```python
from build123d import *

# Parameters (mm, degrees)
SKETCH1_R           = 2.38125
BOSS_EXTRUDE1_DEPTH = 1.5875
SKETCH2_R           = 3.96875
BOSS_EXTRUDE2_DEPTH = 1.5875


with BuildPart() as part:
    # Sketch1 → Boss-Extrude1 (new body)
    with BuildSketch(Plane(origin=(0, 0, 0), x_dir=(1, 0, 0), z_dir=(0, 1, 0))):
        with BuildLine():
            Line((3.96875, 0), (3.921336464, 0.61163461))
            ThreePointArc((3.921336464, 0.61163461), (0, 3.96875), (-3.921336464, 0.61163461))
            Line((-3.921336464, 0.61163461), (-3.96875, 0))
            ThreePointArc((-3.96875, 0), (0, -3.96875), (3.96875, 0))
        make_face()
        with BuildLine():
            Line((3.921336464, 0.61163461), (2.38125, 20.47875))
            ThreePointArc((2.38125, 20.47875), (0, 18.0975), (-2.38125, 20.47875))
            Line((-2.38125, 20.47875), (-3.921336464, 0.61163461))
            ThreePointArc((-3.921336464, 0.61163461), (0, 3.96875), (3.921336464, 0.61163461))
        make_face()
        with Locations((0, 20.47875)):
            Circle(SKETCH1_R)
    extrude(amount=BOSS_EXTRUDE1_DEPTH)

    # Sketch2 → Boss-Extrude2 (add)
    with BuildSketch(Plane(origin=(0, 1.5875, 0), x_dir=(1, 0, 0), z_dir=(0, 1, 0))):
        with Locations(Location((0, 0, 0), (0, 0, 8.865336937))):
            Circle(SKETCH2_R)
    extrude(amount=BOSS_EXTRUDE2_DEPTH)


solid = part.part
```
Geometry: final body of the model. Coordinates: model frame, mm. A direction names the side the tool comes from. Round coordinates to 2 decimals unless told otherwise and drop trailing zeros. Loops run counter-clockwise (first coordinate to the right, second up) from the corner with the lowest first, then second, coordinate; pieces in that order, holes last. Notation, with made-up numbers: (31.25, 43.25) -> (90.25, 43.25) arc R13 ccw to (90.25, 59.25) -> close; hole circle Ø5 at (89.25, -6.75). An arc over 180 degrees is marked (long way). Write each question's results on one line, items separated by ' | '.
Item 1: Set-up query: faces 1 (the face through (-0.25, 1.92, 3.96)), 2 (the face through (0, 3.175, 0)). Return all of +Z, -Z, +X, -X, +Y, -Y with unobstructed straight access to the full face (end or side cutting, diameter ignored); none if empty.
Answers below:
face 1: +Y | face 2: +Z, -Z, +X, -X, +Y
Item 2: Cut plane D-D on y = 2.7. Return the cut outline in (x, z), and give its area (3 significant figures).
Answers below:
outline: circle Ø7.94 at (0, 0) | area: 49.5 mm²
Item 3: Pin query (flat end, axial travel): pin 1 Ø4 at (x, z) = (1.5, -16) entering from +Y; pin 2 Ø1 at (x, y) = (-1, 1) entering from -Z; pin 3 Ø1 at (y, z) = (2, -9) entering from +X. Return the tip coordinate at first contact, or that it passes through.
Answers below:
pin 1: stops at y = 1.59 | pin 2: stops at z = -22.81 | pin 3: stops at x = 3.29
Item 4: Line query: probe 1 along Y at (x, z) = (-0.25, -6.5); probe 2 along Z at (x, y) = (3.5, 2.95); probe 3 along Z at (x, y) = (-0.75, 2.6). Output: solid intervals per line, ascending. Write a range as [from, to].
Answers below:
probe 1: y = [0, 1.59] | probe 2: z = [-1.87, 1.87] | probe 3: z = [-3.9, 3.9]
Item 5: Cut plane C-C on x = 0. Return the cut outline in (y, z) (1 decimal), and give its area (3 significant figures).
Answers below:
outline: (0, -22.9) -> (1.6, -22.9) -> (1.6, -4) -> (3.2, -4) -> (3.2, 4) -> (0, 4) -> close | area: 55.2 mm²
Item 6: Cut plane A-A on y = 0.45. Return the cut outline in (x, z).
Answers below:
outline: (-3.97, 0) -> (-2.38, -20.48) arc R2.38 ccw to (2.38, -20.48) -> (3.97, 0) arc R3.97 ccw to start
